Design review of the part shown in the three views and the two pictorial views. Dimensions are in mm from the part's minimum x, y and z. A direction names the side the tool comes from. Give positions to 0.01 mm unless a question says otherwise; leave off trailing zeros. Order: outer loops, then holes, each group sorted by start corner. A loop starts at its lowest first (then second) coordinate and runs counter-clockwise, first axis right, second up.
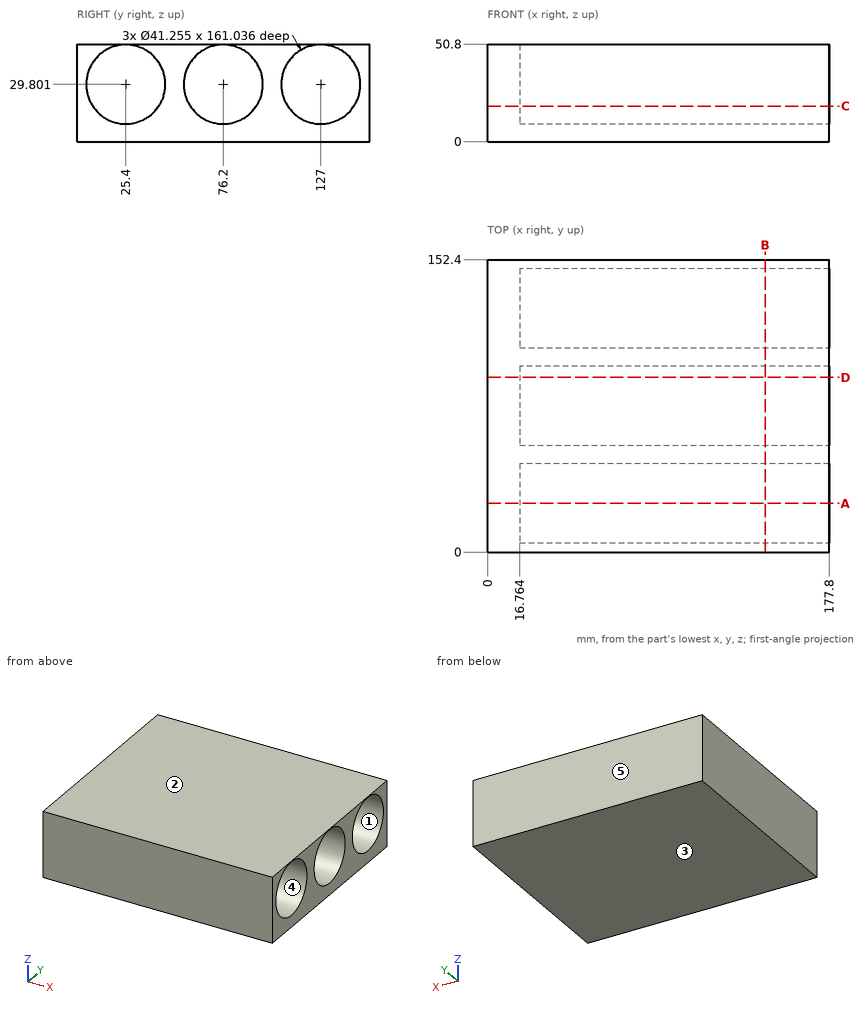
Item 1: Take a section at D-D (y = 91). Give the boundary of the cut face in (x, z).
Values found:
outline: (0, 0) - (177.8, 0) - (177.8, 15.43) - (16.76, 15.43) - (16.76, 44.17) - (177.8, 44.17) - (177.8, 50.8) - (0, 50.8) - close
Item 2: Draft analysis for pull direction Z (two halves, no side actions). For the marked faces 3, 4 and 5, state which applies: released by +Z, released by -Z, zero draft, split by the parting line, or undercut.
Values found:
face 3: released by -Z
face 4: undercut
face 5: zero draft
Item 3: Take a section at B-B (x = 144.5). Give the boundary of the cut face in (y, z) (1 decimal).
Values found:
outline: (0, 0) - (152.4, 0) - (152.4, 50.8) - (0, 50.8) - close; hole circle Ø41.3 at (25.4, 29.8); hole circle Ø41.3 at (76.2, 29.8); hole circle Ø41.3 at (127, 29.8)
Item 4: Take a section at C-C (z = 18.5). Give the boundary of the cut face in (x, y).
Values found:
outline: (0, 0) - (177.8, 0) - (177.8, 8.14) - (16.76, 8.14) - (16.76, 42.66) - (177.8, 42.66) - (177.8, 58.94) - (16.76, 58.94) - (16.76, 93.46) - (177.8, 93.46) - (177.8, 109.74) - (16.76, 109.74) - (16.76, 144.26) - (177.8, 144.26) - (177.8, 152.4) - (0, 152.4) - close
Item 5: For line 1 (Y direction, x = 57, z = 30); line 2 (Z direction, x = 68, y = 25) (1 decimal); line 3 (Y direction, x = 153, z = 48), list the stretches that pass through material, from the lowest coordinate up.
Values found:
line 1: y = 0 to 4.77, 46.03 to 55.57, 96.83 to 106.37, 147.63 to 152.4
line 2: z = 0 to 9.2, 50.4 to 50.8
line 3: y = 0 to 15.69, 35.11 to 66.49, 85.91 to 117.29, 136.71 to 152.4
Item 6: For the marked faces 1 and 2, list the 3-axis set-ups (+Z, -Z, +X, -X, +Y, -Y) from which the entire face can be reached by the end or side of a thin tool; tool diameter is ignored.
Values found:
face 1: +X
face 2: +Z, +X, -X, +Y, -Y
Item 7: Take a section at A-A (y = 25.4). Give the boundary of the cut face in (x, z), and give its area (3 significant figures).
Values found:
outline: (0, 0) - (177.8, 0) - (177.8, 9.17) - (16.76, 9.17) - (16.76, 50.43) - (177.8, 50.43) - (177.8, 50.8) - (0, 50.8) - close
area: 2,390 mm2
Item 8: Clearance check with a flat-ended pin moving along its axis: pin 1 Ø12.5 at (y, z) = (119, 37.5) entering from +X. State where the tip first meets the part, or that it passes through.
Values found:
pin 1: stops at x = 16.76
